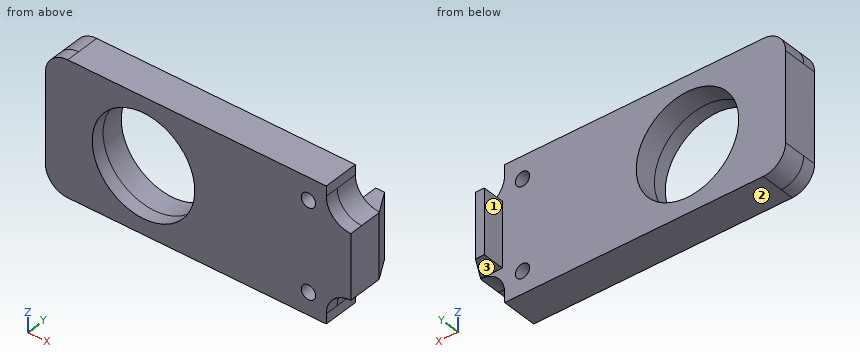
```python
from build123d import *

# Parameters (mm, degrees)
SKETCH1_W           = 63
SKETCH1_H           = 30
SKETCH1_R           = 11.5
BOSS_EXTRUDE1_DEPTH = 5
SKETCH2_R           = 1.6
CUT_EXTRUDE1_DEPTH  = 70.95712973
FILLET1_R           = 5
SKETCH3_W           = 14.5
SKETCH3_H           = 5
BOSS_EXTRUDE2_DEPTH = 0.5
SKETCH4_W           = 14.5
SKETCH4_H           = 10
BOSS_EXTRUDE3_DEPTH = 5
FILLET2_R           = 5.5
SKETCH5_W           = 3.208712153
SKETCH5_H           = 5
CUT_EXTRUDE2_DEPTH  = 76.447001266
CHAMFER1_SIZE       = 5.196152423
CHAMFER1_SIZE_2     = 3
SKETCH6_R           = 1.6
SKETCH6_R_2         = 11.5
BOSS_EXTRUDE4_DEPTH = 3


with BuildPart() as part:
    # Sketch1 → Boss-Extrude1 (new body)
    with BuildSketch(Plane(origin=(0, 0, 0), x_dir=(1, 0, 0), z_dir=(0, 1, 0))):
        with Locations((31.5, 15)):
            Rectangle(SKETCH1_W, SKETCH1_H)
        with Locations(Location((22, 15, 0), (0, 0, 270))):
            Circle(SKETCH1_R, mode=Mode.SUBTRACT)
    extrude(amount=BOSS_EXTRUDE1_DEPTH)

    # Sketch2 → Cut-Extrude1 (cut, through all)
    with BuildSketch(Plane(origin=(0, 5, 0), x_dir=(1, 0, 0), z_dir=(0, 1, 0))):
        with Locations(Location((59, 25, 0), (0, 0, 270))):
            Circle(SKETCH2_R)
        with Locations(Location((59, 5, 0), (0, 0, 270))):
            Circle(SKETCH2_R)
    extrude(amount=-CUT_EXTRUDE1_DEPTH, mode=Mode.SUBTRACT)

    # Fillet1
    fillet1_edges = [part.edges().sort_by_distance(p)[0] for p in [
        (0, 2.5, -30),
        (0, 2.5, 0),
    ]]
    fillet(fillet1_edges, radius=FILLET1_R)

    # Sketch3 → Boss-Extrude2 (add)
    with BuildSketch(Plane(origin=(63, 0, 0), x_dir=(0, 0, -1), z_dir=(1, 0, 0))):
        with Locations((15, 2.5)):
            Rectangle(SKETCH3_W, SKETCH3_H)
    extrude(amount=BOSS_EXTRUDE2_DEPTH)

    # Sketch4 → Boss-Extrude3 (add)
    with BuildSketch(Plane(origin=(63.5, 0, 0), x_dir=(0, 0, -1), z_dir=(1, 0, 0))):
        with Locations((15, 5)):
            Rectangle(SKETCH4_W, SKETCH4_H)
    extrude(amount=BOSS_EXTRUDE3_DEPTH)

    # Fillet2
    # the kernel refuses this fillet: 5.5 mm, written as the material it adds along each edge
    with BuildSketch(Plane(origin=(63, 18.75, -7.75), x_dir=(1, 0, 0), z_dir=(0, -1, 0))) as fillet2_piece_1_section:
        with BuildLine():
            CenterArc((FILLET2_R, FILLET2_R), FILLET2_R, 180, 90)
            Line((0, FILLET2_R), (0, 0))
            Line((0, 0), (FILLET2_R, 0))
        make_face()
    fillet2_piece_1 = extrude(amount=18.75, mode=Mode.PRIVATE)
    fillet2_piece_1 = split(fillet2_piece_1, bisect_by=Plane(origin=(64.81097146, 5, -6.96855226), z_dir=(0, 1, 0)), keep=Keep.TOP, mode=Mode.PRIVATE)
    fillet2_piece_1 = split(fillet2_piece_1, bisect_by=Plane(origin=(64.81097146, 10, -6.96855226), z_dir=(0, -1, 0)), keep=Keep.TOP, mode=Mode.PRIVATE)
    fillet2_piece_1 = split(fillet2_piece_1, bisect_by=Plane(origin=(63.5, 7.5, -6.96855226), z_dir=(1, 0, 0)), keep=Keep.TOP, mode=Mode.PRIVATE)
    add(fillet2_piece_1)
    with BuildSketch(Plane(origin=(63, 5, -7.75), x_dir=(1, 0, 0), z_dir=(0, -1, 0))) as fillet2_piece_2_section:
        with BuildLine():
            CenterArc((FILLET2_R, FILLET2_R), FILLET2_R, 180, 90)
            Line((0, FILLET2_R), (0, 0))
            Line((0, 0), (FILLET2_R, 0))
        make_face()
    fillet2_piece_2 = extrude(amount=5, mode=Mode.PRIVATE)
    fillet2_piece_2 = split(fillet2_piece_2, bisect_by=Plane(origin=(63.5, 2.5, -6.96855226), z_dir=(1, 0, 0)), keep=Keep.TOP, mode=Mode.PRIVATE)
    add(fillet2_piece_2)
    with BuildSketch(Plane(origin=(63, 5, -7.75), x_dir=(1, 0, 0), z_dir=(0, -1, 0))) as fillet2_piece_3_section:
        with BuildLine():
            CenterArc((FILLET2_R, FILLET2_R), FILLET2_R, 180, 90)
            Line((0, FILLET2_R), (0, 0))
            Line((0, 0), (FILLET2_R, 0))
        make_face()
    fillet2_piece_3 = extrude(amount=5, mode=Mode.PRIVATE)
    fillet2_piece_3 = split(fillet2_piece_3, bisect_by=Plane(origin=(63.5, 2.5, -5.619274201), z_dir=(-1, 0, 0)), keep=Keep.TOP, mode=Mode.PRIVATE)
    add(fillet2_piece_3)
    with BuildSketch(Plane(origin=(63, 0, -22.25), x_dir=(0, 0, -1), z_dir=(0, 1, 0))) as fillet2_piece_4_section:
        with BuildLine():
            CenterArc((FILLET2_R, -FILLET2_R), FILLET2_R, 90, 90)
            Line((0, -FILLET2_R), (0, 0))
            Line((0, 0), (FILLET2_R, 0))
        make_face()
    fillet2_piece_4 = extrude(amount=5, mode=Mode.PRIVATE)
    fillet2_piece_4 = split(fillet2_piece_4, bisect_by=Plane(origin=(63.5, 2.5, -24.380725799), z_dir=(-1, 0, 0)), keep=Keep.TOP, mode=Mode.PRIVATE)
    add(fillet2_piece_4)
    with BuildSketch(Plane(origin=(63, 0, -22.25), x_dir=(0, 0, -1), z_dir=(0, 1, 0))) as fillet2_piece_5_section:
        with BuildLine():
            CenterArc((FILLET2_R, -FILLET2_R), FILLET2_R, 90, 90)
            Line((0, -FILLET2_R), (0, 0))
            Line((0, 0), (FILLET2_R, 0))
        make_face()
    fillet2_piece_5 = extrude(amount=5, mode=Mode.PRIVATE)
    fillet2_piece_5 = split(fillet2_piece_5, bisect_by=Plane(origin=(63.5, 2.5, -23.03144774), z_dir=(1, 0, 0)), keep=Keep.TOP, mode=Mode.PRIVATE)
    add(fillet2_piece_5)
    with BuildSketch(Plane(origin=(63, 0, -22.25), x_dir=(0, 0, -1), z_dir=(0, 1, 0))) as fillet2_piece_6_section:
        with BuildLine():
            CenterArc((FILLET2_R, -FILLET2_R), FILLET2_R, 90, 90)
            Line((0, -FILLET2_R), (0, 0))
            Line((0, 0), (FILLET2_R, 0))
        make_face()
    fillet2_piece_6 = extrude(amount=18.75, mode=Mode.PRIVATE)
    fillet2_piece_6 = split(fillet2_piece_6, bisect_by=Plane(origin=(64.81097146, 5, -23.03144774), z_dir=(0, 1, 0)), keep=Keep.TOP, mode=Mode.PRIVATE)
    fillet2_piece_6 = split(fillet2_piece_6, bisect_by=Plane(origin=(64.81097146, 10, -23.03144774), z_dir=(0, -1, 0)), keep=Keep.TOP, mode=Mode.PRIVATE)
    fillet2_piece_6 = split(fillet2_piece_6, bisect_by=Plane(origin=(63.5, 7.5, -23.03144774), z_dir=(1, 0, 0)), keep=Keep.TOP, mode=Mode.PRIVATE)
    add(fillet2_piece_6)

    # Sketch5 → Cut-Extrude2 (cut, through all)
    with BuildSketch(Plane(origin=(68.5, 0, 0), x_dir=(0, 0, -1), z_dir=(1, 0, 0))):
        with Locations((6.145643924, 7.5)):
            Rectangle(SKETCH5_W, SKETCH5_H)
        with Locations((23.854356077, 7.5)):
            Rectangle(SKETCH5_W, SKETCH5_H)
    extrude(amount=-CUT_EXTRUDE2_DEPTH, mode=Mode.SUBTRACT)

    # Chamfer1
    # the kernel refuses this chamfer: 5.196152423, 3 mm, written as the material it takes off along each edge
    with BuildSketch(Plane(origin=(68.5, 10, -35.692891912), x_dir=(0.01932676561270102, -0.9998132206222079, 0), z_dir=(0, 0, 1))) as chamfer1_piece_1:
        Polygon((CHAMFER1_SIZE * 0.999813220566, -CHAMFER1_SIZE * 0.0193267656116), (-CHAMFER1_SIZE_2 * 0.0193267656127, -CHAMFER1_SIZE_2 * 0.999813220622), (0, 0), align=None)
    extrude(amount=41.385783824, mode=Mode.SUBTRACT)

    # Sketch6 → Boss-Extrude4 (add)
    with BuildSketch(Plane.XZ):
        with BuildLine():
            Line((63, -2.25), (63, 0))
            Line((63, 0), (5, 0))
            ThreePointArc((5, 0), (1.464466094, -1.464466094), (0, -5))
            Line((0, -5), (0, -25))
            ThreePointArc((0, -25), (1.464466094, -28.535533906), (5, -30))
            Line((5, -30), (63, -30))
            Line((63, -30), (63, -27.75))
            ThreePointArc((63, -27.75), (64.610912703, -23.860912703), (68.5, -22.25))
            Line((68.5, -22.25), (68.5, -7.75))
            ThreePointArc((68.5, -7.75), (64.610912703, -6.139087297), (63, -2.25))
        make_face()
        with Locations(Location((59, -5, 0), (0, 0, 90))):
            Circle(SKETCH6_R, mode=Mode.SUBTRACT)
        with Locations(Location((22, -15, 0), (0, 0, 270))):
            Circle(SKETCH6_R_2, mode=Mode.SUBTRACT)
        with Locations(Location((59, -25, 0), (0, 0, 90))):
            Circle(SKETCH6_R, mode=Mode.SUBTRACT)
    extrude(amount=BOSS_EXTRUDE4_DEPTH)


solid = part.part
```
For this review, take the finished solid that the model builds, in its own axes (mm). Face numbers are marked on the shaded views. A direction names the side the tool comes from. Round coordinates to 2 decimals unless told otherwise and drop trailing zeros. Write each loop counter-clockwise with the first axis right and the second up, starting at its lowest first coordinate (ties: lowest second). Pieces come first, ordered by that corner, then holes. Notation, with made-up numbers: (85.25, 76.25) -> (95.25, 76.25) arc R21 ccw to (95.25, 107.25) -> close; hole circle Ø8 at (0, 28.5). An arc over 180 degrees is marked (long way). Use one line per item in the form item = value.
1) Take a section at C-C, the plane y = 0.75. Write out the cut boundary in (x, z).
Found:
outline = (0, -25) arc R5 ccw to (5, -30) -> (63, -30) -> (63, -27.75) arc R5.5 cw to (68.5, -22.25) -> (68.5, -7.75) arc R5.5 cw to (63, -2.25) -> (63, 0) -> (5, 0) arc R5 ccw to (0, -5) -> close; hole circle Ø23 at (22, -15); hole circle Ø3.2 at (59, -25); hole circle Ø3.2 at (59, -5)
2) Take a section at B-B, the plane z = -15. Write out the cut boundary in (x, y), and give its area (3 significant figures).
Found:
outline = (0, -3) -> (10.5, -3) -> (10.5, 5) -> (0, 5) -> close; (33.5, -3) -> (68.5, -3) -> (68.5, 4.8) -> (65.5, 10) -> (63.5, 10) -> (63.5, 5) -> (33.5, 5) -> close
area = 381 mm2
3) Take a section at A-A, the plane x = 22. Write out the cut boundary in (y, z).
Found:
outline = (-3, -30) -> (5, -30) -> (5, -26.5) -> (-3, -26.5) -> close; (-3, -3.5) -> (5, -3.5) -> (5, 0) -> (-3, 0) -> close
4) Tool access review of the marked faces 1, 2 and 3: name each direction out of +Z, -Z, +X, -X, +Y, -Y from which nothing blocks a thin tool from reaching the whole face with its end or side.
Found:
face_1 = +Z, -Z, -X, +Y
face_2 = -Z, +X, -X, +Y, -Y
face_3 = -Z, +X, -X, +Y
5) To check wall thickness, follow L1, parallel to Z at x = 59, y = -0.9; L2, parallel to X at y = -0.95, z = -15; L3, parallel to X at y = 1.75, z = -25. State the ranges of each line that lie inside material, in increasing order. Write a range as from..to.
Found:
L1 = -30..-26.6, -23.4..-6.6, -3.4..0
L2 = 0..10.5, 33.5..68.5
L3 = 0..16.32, 27.68..57.4, 60.6..63.74
6) Take a section at D-D, the plane x = 59. Write out the cut boundary in (y, z).
Found:
outline = (-3, -30) -> (5, -30) -> (5, -26.6) -> (-3, -26.6) -> close; (-3, -23.4) -> (5, -23.4) -> (5, -6.6) -> (-3, -6.6) -> close; (-3, -3.4) -> (5, -3.4) -> (5, 0) -> (-3, 0) -> close
7) Clearance check with flat-ended pins moving along their axes: pin 1 (5 mm diameter, centred on x = 59, z = -5, fed in from -Y); pin 2 (1.8 mm diameter, centred on y = 1, z = -1.5, fed in from +X); pin 3 (2 mm diameter, centred on x = 11, z = -23.5, fed in from +Y); pin 4 (1.5 mm diameter, centred on x = 66.5, y = 7.5, fed in from +Z). State where each tip first meets the part, or that it passes through.
Found:
pin_1 = -3
pin_2 = 63
pin_3 = 5
pin_4 = -7.75
